Study the drawing (mm; zero at the part's minimum x, y, z) and answer. A direction names the side the tool comes from. Round coordinates to 2 decimals unless told otherwise and drop trailing zeros. Loops run counter-clockwise (first coordinate to the right, second up) from the corner with the lowest first, then second, coordinate; pieces in that order, holes last. Notation, with made-up numbers: (41.5, -39) -> (59.5, -39) arc R8 cw to (59.5, -34) -> close; hole circle Ø10 at (59, 65). An arc over 180 degrees is marked (long way). Use one line per item in the form item = value.
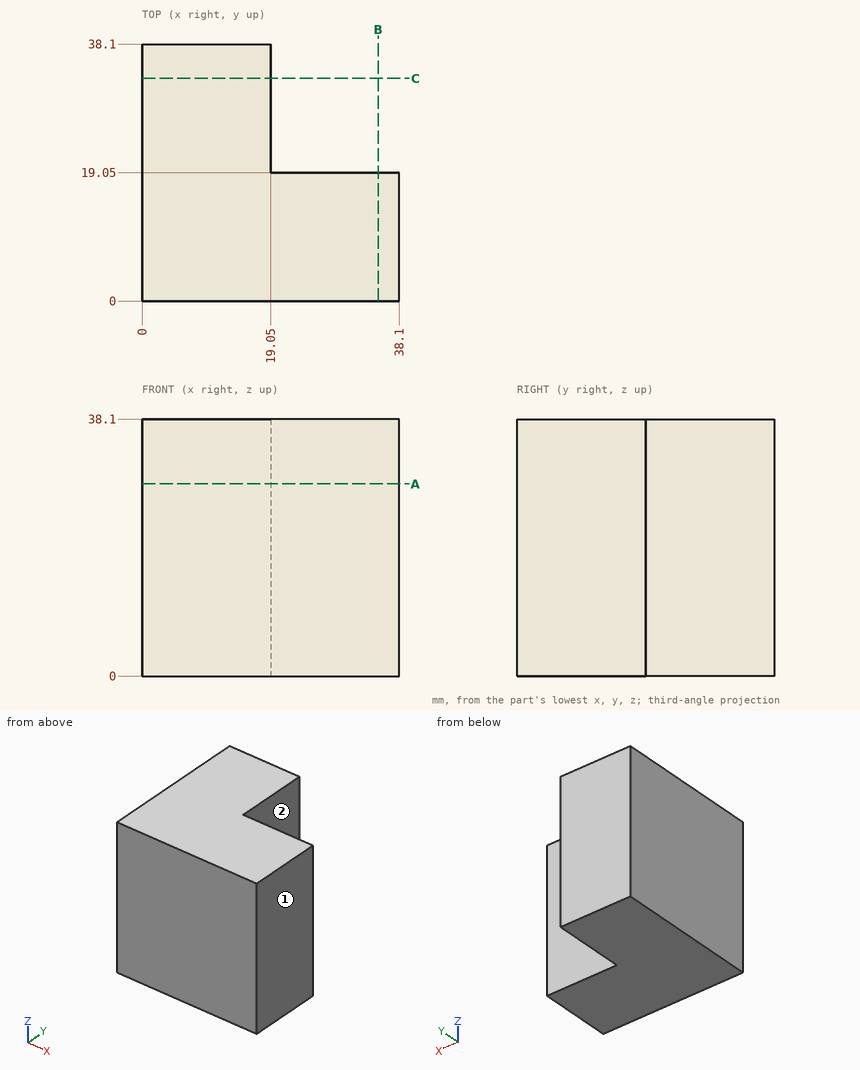
(1) Consider L1, parallel to X at y = 23, z = 35. Determine where the line is inside the solid, lowest interval first.
Completed:
L1 = 0 to 19.05
(2) Given P1, Ø9.5, axis at x = 27, z = 10, coming from the +Y side; P2, Ø9.5, axis at y = 29.5, z = 16, coming from the +X side, each flat-ended and moving along its own axis, determine where each tip first touches the part or whether it passes through.
Completed:
P1 = 19.05
P2 = 19.05
(3) Find section B-B, the plane x = 35. Write down the section's boundary in (y, z), then the cut area to 3 significant figures.
Completed:
outline = (0, 0) -> (19.05, 0) -> (19.05, 38.1) -> (0, 38.1) -> close
area = 726 mm2
(4) For the marked faces 1 and 2, determine the directions among +Z, -Z, +X, -X, +Y, -Y from which every point of the face is accessible in a straight line to the end or side of a thin tool.
Completed:
face_1 = +Z, -Z, +X, +Y, -Y
face_2 = +Z, -Z, +X, +Y
(5) Find section A-A, the plane z = 28.5. Write down the section's boundary in (x, y), then the cut area to 3 significant figures.
Completed:
outline = (0, 0) -> (38.1, 0) -> (38.1, 19.05) -> (19.05, 19.05) -> (19.05, 38.1) -> (0, 38.1) -> close
area = 1,090 mm2
